Design review of the part built by this model. Coordinates are the model's own, in mm. A direction names the side the tool comes from. Coordinates: 2 decimals unless noted, no trailing zeros. Loops run counter-clockwise (first coordinate to the right, second up) from the corner with the lowest first, then second, coordinate; pieces in that order, holes last. Notation, with made-up numbers: (56, -14.5) -> (77, -14.5) arc R34 cw to (77, 21.5) -> close; hole circle Ø3 at (-5.75, 73). An arc over 180 degrees is marked (long way). Use a Markdown table: item, result. Add a question column.
Q1. Clearance check with flat-ended pins moving along their axes: pin 1 Ø3.5 at (x, y) = (0, 0) entering from +Z; pin 2 Ø1.5 at (x, z) = (1.5, 12.5) entering from -Y; pin 3 Ø2 at (x, z) = (3, 15.5) entering from -Y. State where each tip first meets the part, or that it passes through.
Q2. Take a section at C-C on y = -3.25. Write out the cut boundary in (x, z).
Q3. For faces 1 (the face through (2, 0, 5)), 2 (the face through (-2, -1, 0)), 3 (the face through (2, 0, 45)), list the 3-axis set-ups (+Z, -Z, +X, -X, +Y, -Y) from which the entire face can be reached by the end or side of a thin tool; tool diameter is ignored.
Q4. Take a section at A-A on z = 9.5. Write out the cut boundary in (x, y).
Q5. Draft analysis for pull direction Z (two halves, no side actions). For faces 4 (the face through (-0.867, 3.905, 24.65)), 5 (the face through (0.104, 0.331, 10.993)), 6 (the face through (-2, -1, 50)), state which applies: pulls with the +Z half, pulls with the -Z half, needs draft (parallel to the pull), parting line crosses it, or undercut.
Q6. Take a section at B-B on z = 26.5. Write out the cut boundary in (x, y).
Q7. For probe 1 along Y at (x, z) = (0, 43.5); probe 2 along Y at (x, z) = (1.75, 7); probe 3 along X at (y, z) = (-0.25, 21.5), list the stretches that pass through material, from the lowest coordinate up.
Q8. Take a section at D-D on x = 2.75. Write out the cut boundary in (y, z), plus the area to 3 significant figures.
Autodesk Inventor part; units mm, degrees
ref_plane "YZ Plane" through (0, 0, 0) normal (1, 0, 0) x (0, 1, 0)
ref_plane "XZ Plane" through (0, 0, 0) normal (0, 1, 0) x (-1, 0, 0)
ref_plane "XY Plane" through (0, 0, 0) normal (0, 0, 1) x (1, 0, 0)
sketch "Esquisse2" plane through (0, 0, 0) normal (0, 0, 1) x (1, 0, 0)
  circle A0 centre (0, 0) radius 4
  dimension "d4" = 8
extrude "Extrusion2" add sketch "Esquisse2" along normal blind 50
hole "Perçage1" at (0, 0, 50) direction (0, 0, -1) diameter 4 depth 10 tip angle 118
hole "Perçage2" at (0, 0, 0) direction (0, 0, 1) diameter 4 depth 10 tip angle 118
thread "Filetage1"
thread "Filetage2"
properties part number "Tube-4mm" material "Aluminium 6061"
Answer list:
| question | item | result |
|---|---|---|
| 1 | pin 1 | z = 39.85 |
| 1 | pin 2 | y = -3.93 |
| 1 | pin 3 | y = -3.46 |
| 2 | outline | (-2.33, 0) -> (2.33, 0) -> (2.33, 50) -> (-2.33, 50) -> close |
| 3 | face 1 | -Z |
| 3 | face 2 | -Z, +X, -X, +Y, -Y |
| 3 | face 3 | +Z |
| 4 | outline | circle Ø8 at (0, 0); hole circle Ø4 at (0, 0) |
| 5 | face 4 | needs draft |
| 5 | face 5 | pulls with the -Z half |
| 5 | face 6 | pulls with the +Z half |
| 6 | outline | circle Ø8 at (0, 0) |
| 7 | probe 1 | -4 to -2, 2 to 4 |
| 7 | probe 2 | -3.6 to -0.97, 0.97 to 3.6 |
| 7 | probe 3 | -3.99 to 3.99 |
| 8 | outline | (-2.9, 0) -> (2.9, 0) -> (2.9, 50) -> (-2.9, 50) -> close |
| 8 | area | 290 mm² |
